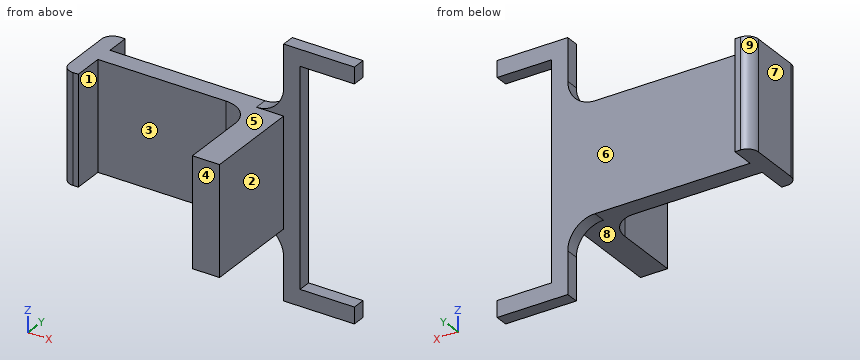
```python
from build123d import *

# Parameters (mm, degrees)
SKETCH1_W           = 33.5
SKETCH1_H           = 20
BOSS_EXTRUDE1_DEPTH = 2.4
BOSS_EXTRUDE2_DEPTH = 10
FILLET1_R           = 5
FILLET2_R           = 5
FILLET3_R           = 2


with BuildPart() as part:
    # Sketch1 → Boss-Extrude1 (new body)
    with BuildSketch(Plane(origin=(0, 0, 0), x_dir=(1, 0, 0), z_dir=(0, 1, 0))):
        with Locations((-29.75, 0)):
            Rectangle(SKETCH1_W, SKETCH1_H)
        Polygon((-10, -19.75), (-10, 19.75), (0, 19.75), (0, 22.75), (-13, 22.75), (-13, -22.75), (0, -22.75), (0, -19.75), align=None)
    extrude(amount=-BOSS_EXTRUDE1_DEPTH)

    # Sketch3 → Boss-Extrude2 (add, symmetric)
    with BuildSketch(Plane.XY):
        Polygon((-13, -2.4), (-13, -20.38), (-18, -20.38), (-18, -3.38), (-46.5, -3.38), (-46.5, -8.875), (-49.5, -8.875), (-49.5, 4.25), (-46.5, 4.25), (-46.5, -2.4), align=None)
    extrude(amount=BOSS_EXTRUDE2_DEPTH, both=True)

    # Fillet1
    fillet1_edges = [part.edges().sort_by_distance(p)[0] for p in [
        (-13, -1.2, -10),
        (-13, -1.2, 10),
    ]]
    fillet(fillet1_edges, radius=FILLET1_R)

    # Fillet2
    fillet2_edges = [part.edges().sort_by_distance(p)[0] for p in [
        (-18, -3.38, 0),
    ]]
    fillet(fillet2_edges, radius=FILLET2_R)

    # Fillet3
    fillet3_edges = [part.edges().sort_by_distance(p)[0] for p in [
        (-49.5, 4.25, 0),
        (-49.5, -8.875, 0),
    ]]
    fillet(fillet3_edges, radius=FILLET3_R)


solid = part.part
```
Could you check a few things on this model? Use its own coordinates, in mm. Face numbers are marked on the shaded views. A direction names the side the tool comes from. Give positions to 0.01 mm unless a question says otherwise; leave off trailing zeros. Loops run counter-clockwise (first coordinate to the right, second up) from the corner with the lowest first, then second, coordinate; pieces in that order, holes last. Notation, with made-up numbers: (-23, -9.75) - (-3, -9.75) arc R20 ccw to (-3, 22.25) - close; hole circle Ø4 at (14.5, -4.75). An arc over 180 degrees is marked (long way). Answer in a Markdown table with one row per item. Add a question column.
Q1. If we section it at B-B (y = -1.25): List the corners of the cut face in (x, z) for me, plus the area to 3 significant figures.
Q2. If we section it at C-C (x = -17): List the corners of the cut face in (y, z) for me.
Q3. For pin 1 (14.5 mm diameter, centred on y = -16, z = 3.5, fed in from +X); pin 2 (0.7 mm diameter, centred on y = -1.5, z = 6.5, fed in from +X); pin 3 (12.5 mm diameter, centred on x = -29, y = -2.5, fed in from +Z), each with a flat end and sliding along its axis, tell me the tip position at first contact or that it passes through.
Q4. Please list where these lines run through material, in increasing order: L1, parallel to X at y = -13.75, z = 6.5; L2, parallel to Y at x = -42, z = -0.5; L3, parallel to X at y = -2.25, z = 21. Write a range as from..to.
Q5. If we section it at A-A (z = -4.5): List the corners of the cut face in (x, y) for me (3 decimals), plus the area to 3 significant figures.
Q6. If we section it at D-D (z = -12): List the corners of the cut face in (x, y) for me, plus the area to 3 significant figures.
Q7. Which directions (+Z, -Z, +X, -X, +Y, -Y) give clear straight access to the entire face, cutting with the end or side of a thin tool? Please do the marked faces 5, 6, 7, 8 and 9.
Q8. We'd pull the mould along X, two halves only. Please class the marked faces 1, 2, 3 and 4: +X half, -X half, draft (parallel to the pull), parting line (faces both ways), or undercut.
The answers:
| question | item | result |
|---|---|---|
| 1 | outline | (-49.5, -10) - (-18, -10) arc R5 cw to (-13, -15) - (-13, -22.75) - (0, -22.75) - (0, -19.75) - (-10, -19.75) - (-10, 19.75) - (0, 19.75) - (0, 22.75) - (-13, 22.75) - (-13, 15) arc R5 cw to (-18, 10) - (-49.5, 10) - close |
| 1 | area | 937 mm^2 |
| 2 | outline | (-20.38, -10) - (-2.4, -10) - (-2.4, -10.1) - (0, -10.1) - (0, 10.1) - (-2.4, 10.1) - (-2.4, 10) - (-20.38, 10) - close |
| 3 | pin 1 | stops at x = -13 |
| 3 | pin 2 | stops at x = -10 |
| 3 | pin 3 | stops at z = 10 |
| 4 | L1 | x = -18..-13 |
| 4 | L2 | y = -3.38..0 |
| 4 | L3 | x = -13..0 |
| 5 | outline | (-49.5, -6.875) arc R2 ccw to (-47.5, -8.875) - (-46.5, -8.875) - (-46.5, -3.38) - (-23, -3.38) arc R5 cw to (-18, -8.38) - (-18, -20.38) - (-13, -20.38) - (-13, -2.4) - (-10, -2.4) - (-10, 0) - (-46.5, 0) - (-46.5, 4.25) - (-47.5, 4.25) arc R2 ccw to (-49.5, 2.25) - close |
| 5 | area | 248 mm^2 |
| 6 | outline | (-14, -2.4) - (-10, -2.4) - (-10, 0) - (-14, 0) - close |
| 6 | area | 9.60 mm^2 |
| 7 | face 5 | +Z, -X, -Y |
| 7 | face 6 | +Z, -Z, +X, +Y |
| 7 | face 7 | +Z, -Z, -X, +Y, -Y |
| 7 | face 8 | -Z, -X, -Y |
| 7 | face 9 | +Z, -Z, -X, +Y |
| 8 | face 1 | undercut |
| 8 | face 2 | +X half |
| 8 | face 3 | undercut |
| 8 | face 4 | draft |
